```python
from build123d import *

# Parameters (mm, degrees)
ESQUISSE1_R        = 3.4
BOSS_EXTRU_1_DEPTH = 832


with BuildPart() as part:
    # Esquisse1 → Boss.-Extru.1 (new body)
    with BuildSketch(Plane(origin=(0, 0, -30), x_dir=(-1, 0, 0), z_dir=(0, 0, -1))):
        with BuildLine():
            Line((-4.5, 15), (-4.5, 13.5))
            ThreePointArc((-4.5, 13.5), (-4.353553391, 13.146446609), (-4, 13))
            Line((-4, 13), (-2.5, 13))
            ThreePointArc((-2.5, 13), (-2.146446609, 12.853553391), (-2, 12.5))
            ThreePointArc((-2, 12.5), (-2.732233047, 10.732233047), (-4.5, 10))
            Line((-4.5, 10), (-5.807611845, 10))
            ThreePointArc((-5.807611845, 10), (-7.721029006, 10.380602337), (-9.343145751, 11.464466094))
            Line((-9.343145751, 11.464466094), (-10.785533906, 12.906854249))
            ThreePointArc((-10.785533906, 12.906854249), (-11.869397663, 14.528970994), (-12.25, 16.442388155))
            Line((-12.25, 16.442388155), (-12.25, 23.557611845))
            ThreePointArc((-12.25, 23.557611845), (-11.869397663, 25.471029006), (-10.785533906, 27.093145751))
            Line((-10.785533906, 27.093145751), (-9.343145751, 28.535533906))
            ThreePointArc((-9.343145751, 28.535533906), (-7.721029006, 29.619397663), (-5.807611845, 30))
            Line((-5.807611845, 30), (-4.5, 30))
            ThreePointArc((-4.5, 30), (-2.732233047, 29.267766953), (-2, 27.5))
            ThreePointArc((-2, 27.5), (-2.146446609, 27.146446609), (-2.5, 27))
            Line((-2.5, 27), (-4, 27))
            ThreePointArc((-4, 27), (-4.353553391, 26.853553391), (-4.5, 26.5))
            Line((-4.5, 26.5), (-4.5, 25))
            ThreePointArc((-4.5, 25), (-4.207106781, 24.292893219), (-3.5, 24))
            Line((-3.5, 24), (-1.5, 24))
            ThreePointArc((-1.5, 24), (-0.439339828, 24.439339828), (0, 25.5))
            Line((0, 25.5), (0, 36))
            ThreePointArc((0, 36), (-1.171572875, 38.828427125), (-4, 40))
            Line((-4, 40), (-14.5, 40))
            ThreePointArc((-14.5, 40), (-15.560660172, 39.560660172), (-16, 38.5))
            Line((-16, 38.5), (-16, 36.5))
            ThreePointArc((-16, 36.5), (-15.707106781, 35.792893219), (-15, 35.5))
            Line((-15, 35.5), (-13.5, 35.5))
            ThreePointArc((-13.5, 35.5), (-13.146446609, 35.646446609), (-13, 36))
            Line((-13, 36), (-13, 37.5))
            ThreePointArc((-13, 37.5), (-12.853553391, 37.853553391), (-12.5, 38))
            ThreePointArc((-12.5, 38), (-10.732233047, 37.267766953), (-10, 35.5))
            Line((-10, 35.5), (-10, 34.192388155))
            ThreePointArc((-10, 34.192388155), (-10.380602337, 32.278970994), (-11.464466094, 30.656854249))
            Line((-11.464466094, 30.656854249), (-12.906854249, 29.214466094))
            ThreePointArc((-12.906854249, 29.214466094), (-14.528970994, 28.130602337), (-16.442388155, 27.75))
            Line((-16.442388155, 27.75), (-23.557611845, 27.75))
            ThreePointArc((-23.557611845, 27.75), (-25.471029006, 28.130602337), (-27.093145751, 29.214466094))
            Line((-27.093145751, 29.214466094), (-28.535533906, 30.656854249))
            ThreePointArc((-28.535533906, 30.656854249), (-29.619397663, 32.278970994), (-30, 34.192388155))
            Line((-30, 34.192388155), (-30, 35.5))
            ThreePointArc((-30, 35.5), (-29.267766953, 37.267766953), (-27.5, 38))
            ThreePointArc((-27.5, 38), (-27.146446609, 37.853553391), (-27, 37.5))
            Line((-27, 37.5), (-27, 36))
            ThreePointArc((-27, 36), (-26.853553391, 35.646446609), (-26.5, 35.5))
            Line((-26.5, 35.5), (-25, 35.5))
            ThreePointArc((-25, 35.5), (-24.292893219, 35.792893219), (-24, 36.5))
            Line((-24, 36.5), (-24, 38.5))
            ThreePointArc((-24, 38.5), (-24.439339828, 39.560660172), (-25.5, 40))
            Line((-25.5, 40), (-36, 40))
            ThreePointArc((-36, 40), (-38.828427125, 38.828427125), (-40, 36))
            Line((-40, 36), (-40, 25.5))
            ThreePointArc((-40, 25.5), (-39.560660172, 24.439339828), (-38.5, 24))
            Line((-38.5, 24), (-36.5, 24))
            ThreePointArc((-36.5, 24), (-35.792893219, 24.292893219), (-35.5, 25))
            Line((-35.5, 25), (-35.5, 26.5))
            ThreePointArc((-35.5, 26.5), (-35.646446609, 26.853553391), (-36, 27))
            Line((-36, 27), (-37.5, 27))
            ThreePointArc((-37.5, 27), (-37.853553391, 27.146446609), (-38, 27.5))
            ThreePointArc((-38, 27.5), (-37.267766953, 29.267766953), (-35.5, 30))
            Line((-35.5, 30), (-34.192388155, 30))
            ThreePointArc((-34.192388155, 30), (-32.278970994, 29.619397663), (-30.656854249, 28.535533906))
            Line((-30.656854249, 28.535533906), (-29.214466094, 27.093145751))
            ThreePointArc((-29.214466094, 27.093145751), (-28.130602337, 25.471029006), (-27.75, 23.557611845))
            Line((-27.75, 23.557611845), (-27.75, 16.442388155))
            ThreePointArc((-27.75, 16.442388155), (-28.130602337, 14.528970994), (-29.214466094, 12.906854249))
            Line((-29.214466094, 12.906854249), (-30.656854249, 11.464466094))
            ThreePointArc((-30.656854249, 11.464466094), (-32.278970994, 10.380602337), (-34.192388155, 10))
            Line((-34.192388155, 10), (-35.5, 10))
            ThreePointArc((-35.5, 10), (-37.267766953, 10.732233047), (-38, 12.5))
            ThreePointArc((-38, 12.5), (-37.853553391, 12.853553391), (-37.5, 13))
            Line((-37.5, 13), (-36, 13))
            ThreePointArc((-36, 13), (-35.646446609, 13.146446609), (-35.5, 13.5))
            Line((-35.5, 13.5), (-35.5, 15))
            ThreePointArc((-35.5, 15), (-35.792893219, 15.707106781), (-36.5, 16))
            Line((-36.5, 16), (-38.5, 16))
            ThreePointArc((-38.5, 16), (-39.560660172, 15.560660172), (-40, 14.5))
            Line((-40, 14.5), (-40, 4))
            ThreePointArc((-40, 4), (-38.828427125, 1.171572875), (-36, 0))
            Line((-36, 0), (-25.5, 0))
            ThreePointArc((-25.5, 0), (-24.439339828, 0.439339828), (-24, 1.5))
            Line((-24, 1.5), (-24, 3.5))
            ThreePointArc((-24, 3.5), (-24.292893219, 4.207106781), (-25, 4.5))
            Line((-25, 4.5), (-26.5, 4.5))
            ThreePointArc((-26.5, 4.5), (-26.853553391, 4.353553391), (-27, 4))
            Line((-27, 4), (-27, 2.5))
            ThreePointArc((-27, 2.5), (-27.146446609, 2.146446609), (-27.5, 2))
            ThreePointArc((-27.5, 2), (-29.267766953, 2.732233047), (-30, 4.5))
            Line((-30, 4.5), (-30, 5.807611845))
            ThreePointArc((-30, 5.807611845), (-29.619397663, 7.721029006), (-28.535533906, 9.343145751))
            Line((-28.535533906, 9.343145751), (-27.093145751, 10.785533906))
            ThreePointArc((-27.093145751, 10.785533906), (-25.471029006, 11.869397663), (-23.557611845, 12.25))
            Line((-23.557611845, 12.25), (-16.442388155, 12.25))
            ThreePointArc((-16.442388155, 12.25), (-14.528970994, 11.869397663), (-12.906854249, 10.785533906))
            Line((-12.906854249, 10.785533906), (-11.464466094, 9.343145751))
            ThreePointArc((-11.464466094, 9.343145751), (-10.380602337, 7.721029006), (-10, 5.807611845))
            Line((-10, 5.807611845), (-10, 4.5))
            ThreePointArc((-10, 4.5), (-10.732233047, 2.732233047), (-12.5, 2))
            ThreePointArc((-12.5, 2), (-12.853553391, 2.146446609), (-13, 2.5))
            Line((-13, 2.5), (-13, 4))
            ThreePointArc((-13, 4), (-13.146446609, 4.353553391), (-13.5, 4.5))
            Line((-13.5, 4.5), (-15, 4.5))
            ThreePointArc((-15, 4.5), (-15.707106781, 4.207106781), (-16, 3.5))
            Line((-16, 3.5), (-16, 1.5))
            ThreePointArc((-16, 1.5), (-15.560660172, 0.439339828), (-14.5, 0))
            Line((-14.5, 0), (-4, 0))
            ThreePointArc((-4, 0), (-1.171572875, 1.171572875), (0, 4))
            Line((0, 4), (0, 14.5))
            ThreePointArc((0, 14.5), (-0.439339828, 15.560660172), (-1.5, 16))
            Line((-1.5, 16), (-3.5, 16))
            ThreePointArc((-3.5, 16), (-4.207106781, 15.707106781), (-4.5, 15))
        make_face()
        with Locations((-20, 20)):
            Circle(ESQUISSE1_R, mode=Mode.SUBTRACT)
        with BuildLine():
            Line((-4, 1.8), (-7.7, 1.8))
            ThreePointArc((-7.7, 1.8), (-8.053553391, 1.946446609), (-8.2, 2.3))
            Line((-8.2, 2.3), (-8.2, 7.7))
            ThreePointArc((-8.2, 7.7), (-8.053553391, 8.053553391), (-7.7, 8.2))
            Line((-7.7, 8.2), (-2.3, 8.2))
            ThreePointArc((-2.3, 8.2), (-1.946446609, 8.053553391), (-1.8, 7.7))
            Line((-1.8, 7.7), (-1.8, 4))
            ThreePointArc((-1.8, 4), (-2.444365081, 2.444365081), (-4, 1.8))
        make_face(mode=Mode.SUBTRACT)
        with BuildLine():
            Line((-38.2, 4), (-38.2, 7.7))
            ThreePointArc((-38.2, 7.7), (-38.053553391, 8.053553391), (-37.7, 8.2))
            Line((-37.7, 8.2), (-32.3, 8.2))
            ThreePointArc((-32.3, 8.2), (-31.946446609, 8.053553391), (-31.8, 7.7))
            Line((-31.8, 7.7), (-31.8, 2.3))
            ThreePointArc((-31.8, 2.3), (-31.946446609, 1.946446609), (-32.3, 1.8))
            Line((-32.3, 1.8), (-36, 1.8))
            ThreePointArc((-36, 1.8), (-37.555634919, 2.444365081), (-38.2, 4))
        make_face(mode=Mode.SUBTRACT)
        with BuildLine():
            Line((-36, 38.2), (-32.3, 38.2))
            ThreePointArc((-32.3, 38.2), (-31.946446609, 38.053553391), (-31.8, 37.7))
            Line((-31.8, 37.7), (-31.8, 32.3))
            ThreePointArc((-31.8, 32.3), (-31.946446609, 31.946446609), (-32.3, 31.8))
            Line((-32.3, 31.8), (-37.7, 31.8))
            ThreePointArc((-37.7, 31.8), (-38.053553391, 31.946446609), (-38.2, 32.3))
            Line((-38.2, 32.3), (-38.2, 36))
            ThreePointArc((-38.2, 36), (-37.555634919, 37.555634919), (-36, 38.2))
        make_face(mode=Mode.SUBTRACT)
        with BuildLine():
            Line((-1.8, 36), (-1.8, 32.3))
            ThreePointArc((-1.8, 32.3), (-1.946446609, 31.946446609), (-2.3, 31.8))
            Line((-2.3, 31.8), (-7.7, 31.8))
            ThreePointArc((-7.7, 31.8), (-8.053553391, 31.946446609), (-8.2, 32.3))
            Line((-8.2, 32.3), (-8.2, 37.7))
            ThreePointArc((-8.2, 37.7), (-8.053553391, 38.053553391), (-7.7, 38.2))
            Line((-7.7, 38.2), (-4, 38.2))
            ThreePointArc((-4, 38.2), (-2.444365081, 37.555634919), (-1.8, 36))
        make_face(mode=Mode.SUBTRACT)
    extrude(amount=-BOSS_EXTRU_1_DEPTH)


solid = part.part
```
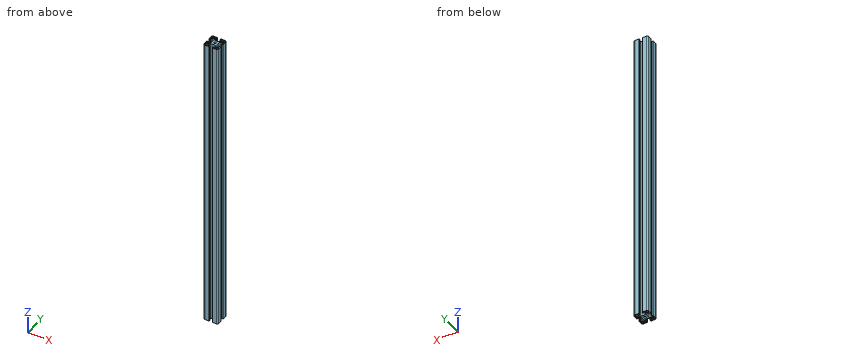
Could you check a few things on this model? Use its own coordinates, in mm. Give positions to 0.01 mm unless a question says otherwise; leave off trailing zeros. Answer in a Markdown table with one row per item. Add a question column.
Q1. For pin 1 (2 mm diameter, centred on y = 18, z = 559.5, fed in from +X); pin 2 (5.5 mm diameter, centred on x = 20, y = 20, fed in from -Z); pin 3 (1 mm diameter, centred on y = 2, z = 220, fed in from -X); pin 4 (0.6 mm diameter, centred on y = 3, z = 354, fed in from +X), each with a flat end and sliding along its axis, tell me the tip position at first contact or that it passes through.
Q2. If we section it at A-A (z = 174.5): State how many separate pieces and enclosed holes the cut face has, plus the area to 3 significant figures.
Q3. Please list where these lines run through material, in increasing order: L1, parallel to Y at x = 33, z = 167; L2, parallel to X at y = 33.5, z = 719. Write a range as from..to.
The answers:
| question | item | result |
|---|---|---|
| 1 | pin 1 | stops at x = 27.75 |
| 1 | pin 2 | passes through |
| 1 | pin 3 | stops at x = 0.29 |
| 1 | pin 4 | stops at x = 39.94 |
| 2 | separate pieces | 1 |
| 2 | enclosed holes | 5 |
| 2 | area | 657 mm^2 |
| 3 | L1 | y = 0..1.8, 8.2..10.14, 29.86..31.8, 38.2..40 |
| 3 | L2 | x = 0..1.8, 8.2..10.05, 29.95..31.8, 38.2..40 |
